from build123d import *

# Parameters (mm, degrees)
SKETCH1_R           = 12.5
SKETCH1_R_2         = 19
BOSS_EXTRUDE1_DEPTH = 150
SKETCH2_W           = 4
SKETCH2_H           = 4
CUT_EXTRUDE1_DEPTH  = 151
CIRPATTERN1_COUNT   = 5


with BuildPart() as part:
    # Sketch1 → Boss-Extrude1 (new body)
    with BuildSketch(Plane.XY):
        with BuildLine():
            ThreePointArc((35.904326013, -18.904326024), (15, 0), (35.904326013, 18.904326024))
            ThreePointArc((35.904326013, 18.904326024), (24.373623204, 24.373623204), (18.904326024, 35.904326013))
            ThreePointArc((18.904326024, 35.904326013), (18.976066432, 34.953363922), (19, 34))
            ThreePointArc((19, 34), (-0.953363922, 15.023933568), (-18.904326024, 35.904326013))
            ThreePointArc((-18.904326024, 35.904326013), (-24.373623204, 24.373623204), (-35.904326013, 18.904326024))
            ThreePointArc((-35.904326013, 18.904326024), (-21.25602484, 14.092235349), (-15, 0))
            ThreePointArc((-15, 0), (-21.25602484, -14.092235349), (-35.904326013, -18.904326024))
            ThreePointArc((-35.904326013, -18.904326024), (-24.373623204, -24.373623204), (-18.904326024, -35.904326013))
            ThreePointArc((-18.904326024, -35.904326013), (-0.953363922, -15.023933568), (19, -34))
            ThreePointArc((19, -34), (18.976066432, -34.953363922), (18.904326024, -35.904326013))
            ThreePointArc((18.904326024, -35.904326013), (24.373623204, -24.373623204), (35.904326013, -18.904326024))
        make_face()
        Circle(SKETCH1_R, mode=Mode.SUBTRACT)
        with Locations((0, 34)):
            Circle(SKETCH1_R_2)
        with Locations((-34, 0)):
            Circle(SKETCH1_R_2)
        with Locations((0, -34)):
            Circle(SKETCH1_R_2)
        with Locations((34, 0)):
            Circle(SKETCH1_R_2)
    extrude(amount=BOSS_EXTRUDE1_DEPTH)

    # Sketch2 → Cut-Extrude1 (cut, through all)
    with BuildSketch(Plane(origin=(0, 0, 0), x_dir=(-1, 0, 0), z_dir=(0, 0, -1))):
        with Locations((12.5, 0)):
            Rectangle(SKETCH2_W, SKETCH2_H)
    cut_extrude1 = extrude(amount=-CUT_EXTRUDE1_DEPTH, mode=Mode.SUBTRACT)

    # CirPattern1: Cut-Extrude1 ×5 about axis
    cirpattern1_axis = Axis((0, 0, 0), (0, 0, 1))
    for i in range(1, CIRPATTERN1_COUNT):
        add(cut_extrude1.rotate(cirpattern1_axis, i * 360 / CIRPATTERN1_COUNT), mode=Mode.SUBTRACT)


solid = part.part
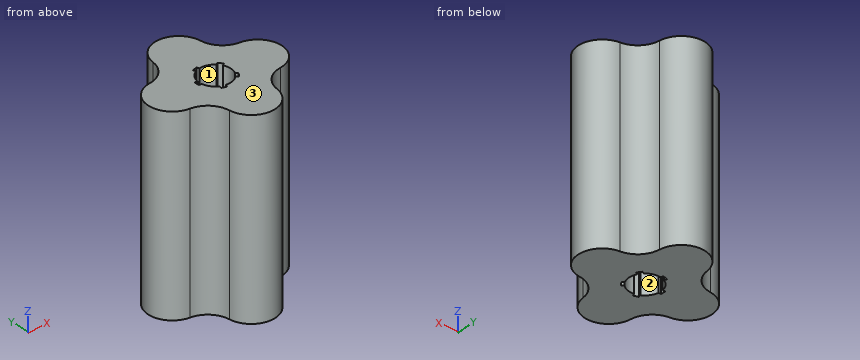
Model file for the job. Use its own axes, mm. Face numbers are marked on the shaded views. Round coordinates to 2 decimals unless told otherwise and drop trailing zeros. Order: outer loops, then holes, each group sorted by start corner. A loop starts at its lowest first (then second) coordinate and runs counter-clockwise, first axis right, second up.
(1) Pull direction Y, two halves, no side cores. Call the marked faces 1, 2 and 3: released by +Y, released by -Y, zero draft, split by the parting line, or undercut.
(2) Band-saw the part on A-A (z = 54). List the corners of the cut face in (x, y), then the cut area to 3 significant figures.
(3) Pin check, flat tips, straight feed: pin 1 (4 mm diameter, centred on y = 35, z = 86, fed in from +X); pin 2 (4.5 mm diameter, centred on y = 1, z = 51, fed in from +X); pin 3 (10 mm diameter, centred on y = -38.5, z = 133, fed in from -X). Stop position of each tip, or through.
(4) Drill centre lines: line 1 (X direction, y = 9, z = 24); line 2 (X direction, y = 11, z = 85.5); line 3 (Y direction, x = 6.5, z = 31.5). Where is each one in solid material? Low to high.
(5) Band-saw the part on B-B (x = 40). List the corners of the cut face in (y, z).
(6) Band-saw the part on C-C (y = 47). List the corners of the cut face in (x, z).
Verdict:
1. face 1: undercut
1. face 2: undercut
1. face 3: zero draft
2. outline: (-35.9, -18.9) arc R19 cw to (-18.9, -35.9) arc R19 ccw to (18.9, -35.9) arc R19 cw to (35.9, -18.9) arc R19 ccw to (35.9, 18.9) arc R19 cw to (18.9, 35.9) arc R19 ccw to (-18.9, 35.9) arc R19 cw to (-35.9, 18.9) arc R19 ccw to start; hole (-14.5, -2) - (-12.34, -2) arc R12.5 ccw to (-5.72, -11.12) - (-6.38, -13.17) - (-2.58, -14.41) - (-1.91, -12.35) arc R12.5 ccw to (8.81, -8.87) - (10.56, -10.14) - (12.91, -6.9) - (11.16, -5.63) arc R12.5 ccw to (11.16, 5.63) - (12.91, 6.9) - (10.56, 10.14) - (8.81, 8.87) arc R12.5 ccw to (-1.91, 12.35) - (-2.58, 14.41) - (-6.38, 13.17) - (-5.72, 11.12) arc R12.5 ccw to (-12.34, 2) - (-14.5, 2) - close
2. area: 5,740 mm2
3. pin 1: stops at x = 19.43
3. pin 2: stops at x = 53
3. pin 3: stops at x = -19.3
4. line 1: x = -50.73 to -8.67, 8.67 to 8.98, 11.38 to 50.73
4. line 2: x = -49.49 to -5.94, 5.94 to 49.49
4. line 3: y = -51.85 to -10.68, 10.68 to 51.85
5. outline: (-18.03, 0) - (18.03, 0) - (18.03, 150) - (-18.03, 150) - close
6. outline: (-13.86, 0) - (13.86, 0) - (13.86, 150) - (-13.86, 150) - close
